The model under review builds one solid part; all positions refer to its coordinate system, in mm. A direction names the side the tool comes from. Coordinates: 2 decimals unless noted, no trailing zeros. Loops run counter-clockwise (first coordinate to the right, second up) from the corner with the lowest first, then second, coordinate; pieces in that order, holes last. Notation, with made-up numbers: (37, -9.5) - (51, -9.5) arc R25 ccw to (51, 13.5) - close; hole circle Ø11 at (-32.75, 68.5). An arc over 180 degrees is marked (long way). Answer in a Markdown table with one row per item. Add a question column.
(1) For P1, Ø6, axis at x = -5, y = 2.5, coming from the -Z side; P2, Ø2, axis at y = -5.5, z = 51, coming from the -X side; P3, Ø5.5, axis at x = -1, z = 11.5, coming from the +Y side; P4, Ø10, axis at x = -3, z = 30.5, coming from the +Y side, all flat-tipped, find the tip position at first contact; note any pin that passes through.
(2) Machinability: for faces 1 (the cylindrical face through (9.014, 2.839, 109.811)), 2 (the cylindrical face through (-1.604, -7.224, 13.903)), 3 (the cylindrical face through (4.57, 7.167, 117.875)), 4 (the flat face through (-8, 4, 72.8)), 5 (the cylindrical face through (-0.05, 6.17, 5.18)), which of the approach directions +Z, -Z, +X, -X, +Y, -Y give a long, thin tool a straight path to every point of the face, cutting with its end or side? Answer none if there is none.
(3) We need section B-B on y = 0. Write out the cut boundary in (x, z).
(4) We need section D-D on z = 13. Write out the cut boundary in (x, y).
(5) Mouldability with a two-part tool opening along Z and no side actions: class faces 6 (the cylindrical face through (9.014, 2.839, 71.761)), 7 (the flat face through (0, 4.9, 16)), 8 (the flat face through (-3, 7, 28.2)) as +Z half, -Z half, draft (parallel to the pull), parting line (faces both ways), or undercut.
(6) We need section C-C on z = 31. Write out the cut boundary in (x, y).
(7) For line 1 along Z through (x, y) = (3, 8.5); line 2 along X through (y, z) = (6.5, 26); line 3 along Z through (x, y) = (-7.5, -0.25), list the stretches that pass through material, from the lowest coordinate up.
(8) We need section A-A on x = 0. Write out the cut boundary in (y, z), plus the area to 3 significant figures.
from build123d import *

# Parameters (mm, degrees)
SKETCH_1_R          = 7.4
EXTRUDE_1_DEPTH     = 28.2
EXTRUDE_START       = 28.2
SKETCH_1_5_R        = 8.5
EXTRUDE_2_DEPTH     = 42.55
EXTRUDE_START_2     = 70.75
SKETCH_1_7_R        = 9.45
EXTRUDE_3_DEPTH     = 2.05
EXTRUDE_START_3     = 108.8
SKETCH_1_8_R        = 9.45
EXTRUDE_4_DEPTH     = 2.05
EXTRUDE_START_4     = 72.8
SKETCH_1_9_R        = 8.5
EXTRUDE_5_DEPTH     = 36
EXTRUDE_START_5     = 110.85
SKETCH_1_10_R       = 8.5
EXTRUDE_6_DEPTH     = 14.25
CUT_EXTRUDE_START   = 7.4
CUT_EXTRUDE_1_DEPTH = 2.5


with BuildPart() as part:
    # Sketch 1 → Extrude 1 (new body)
    with BuildSketch(Plane.XY):
        Circle(SKETCH_1_R)
    extrude(amount=EXTRUDE_1_DEPTH)

    # Sketch 1_5 → Extrude 2 (add)
    with BuildSketch(Plane.XY.offset(EXTRUDE_START)):
        Circle(SKETCH_1_5_R)
    extrude(amount=EXTRUDE_2_DEPTH)

    # Sketch 1_7 → Extrude 3 (add)
    with BuildSketch(Plane.XY.offset(EXTRUDE_START_2)):
        Circle(SKETCH_1_7_R)
    extrude(amount=EXTRUDE_3_DEPTH)



with BuildPart() as body_2:
    # Sketch 1_8 → Extrude 4 (new body)
    with BuildSketch(Plane.XY.offset(EXTRUDE_START_3)):
        Circle(SKETCH_1_8_R)
    extrude(amount=EXTRUDE_4_DEPTH)


with BuildPart() as part_1:
    add(part.part)

    add(body_2.part)  # Extrude 5 merges body 2
    # Sketch 1_9 → Extrude 5 (add)
    with BuildSketch(Plane.XY.offset(EXTRUDE_START_4)):
        Circle(SKETCH_1_9_R)
    extrude(amount=EXTRUDE_5_DEPTH)

    # Sketch 1_10 → Extrude 6 (add)
    with BuildSketch(Plane.XY.offset(EXTRUDE_START_5)):
        Circle(SKETCH_1_10_R)
    extrude(amount=EXTRUDE_6_DEPTH)

    # Sketch 11 → Cut-Extrude 1 (cut)
    with BuildSketch(Plane(origin=(0, 0, 0), x_dir=(1, 0, 0), z_dir=(0, 1, 0)).offset(CUT_EXTRUDE_START)):
        with BuildLine():
            Line((2.5, -7.68), (2.5, -24.22))
            ThreePointArc((2.5, -24.22), (0, -26.72), (-2.5, -24.22))
            Line((-2.5, -24.22), (-2.5, -7.68))
            ThreePointArc((-2.5, -7.68), (0, -5.18), (2.5, -7.68))
        make_face()
    extrude(amount=-CUT_EXTRUDE_1_DEPTH, mode=Mode.SUBTRACT)


solid = part_1.part
Outcome:
| question | item | result |
|---|---|---|
| 1 | P1 | z = 0 |
| 1 | P2 | x = -7.21 |
| 1 | P3 | y = 6.96 |
| 1 | P4 | y = 8.5 |
| 2 | face 1 | +Z, -Z |
| 2 | face 2 | -Z |
| 2 | face 3 | +Z |
| 2 | face 4 | none |
| 2 | face 5 | +Y |
| 3 | outline | (-9.45, 70.75) - (-8.5, 70.75) - (-8.5, 28.2) - (-7.4, 28.2) - (-7.4, 0) - (7.4, 0) - (7.4, 28.2) - (8.5, 28.2) - (8.5, 70.75) - (9.45, 70.75) - (9.45, 72.8) - (8.5, 72.8) - (8.5, 108.8) - (9.45, 108.8) - (9.45, 110.85) - (8.5, 110.85) - (8.5, 125.1) - (-8.5, 125.1) - (-8.5, 110.85) - (-9.45, 110.85) - (-9.45, 108.8) - (-8.5, 108.8) - (-8.5, 72.8) - (-9.45, 72.8) - close |
| 4 | outline | (-2.5, 4.9) - (-2.5, 6.96) arc R7.4 ccw (long way) to (2.5, 6.96) - (2.5, 4.9) - close |
| 5 | face 6 | draft |
| 5 | face 7 | undercut |
| 5 | face 8 | -Z half |
| 6 | outline | circle Ø17 at (0, 0) |
| 7 | line 1 | 70.75 to 72.8, 108.8 to 110.85 |
| 7 | line 2 | -3.54 to -1.76, 1.76 to 3.54 |
| 7 | line 3 | 28.2 to 125.1 |
| 8 | outline | (-9.45, 70.75) - (-8.5, 70.75) - (-8.5, 28.2) - (-7.4, 28.2) - (-7.4, 0) - (7.4, 0) - (7.4, 5.18) - (4.9, 5.18) - (4.9, 26.72) - (7.4, 26.72) - (7.4, 28.2) - (8.5, 28.2) - (8.5, 70.75) - (9.45, 70.75) - (9.45, 72.8) - (8.5, 72.8) - (8.5, 108.8) - (9.45, 108.8) - (9.45, 110.85) - (8.5, 110.85) - (8.5, 125.1) - (-8.5, 125.1) - (-8.5, 110.85) - (-9.45, 110.85) - (-9.45, 108.8) - (-8.5, 108.8) - (-8.5, 72.8) - (-9.45, 72.8) - close |
| 8 | area | 2,020 mm² |
